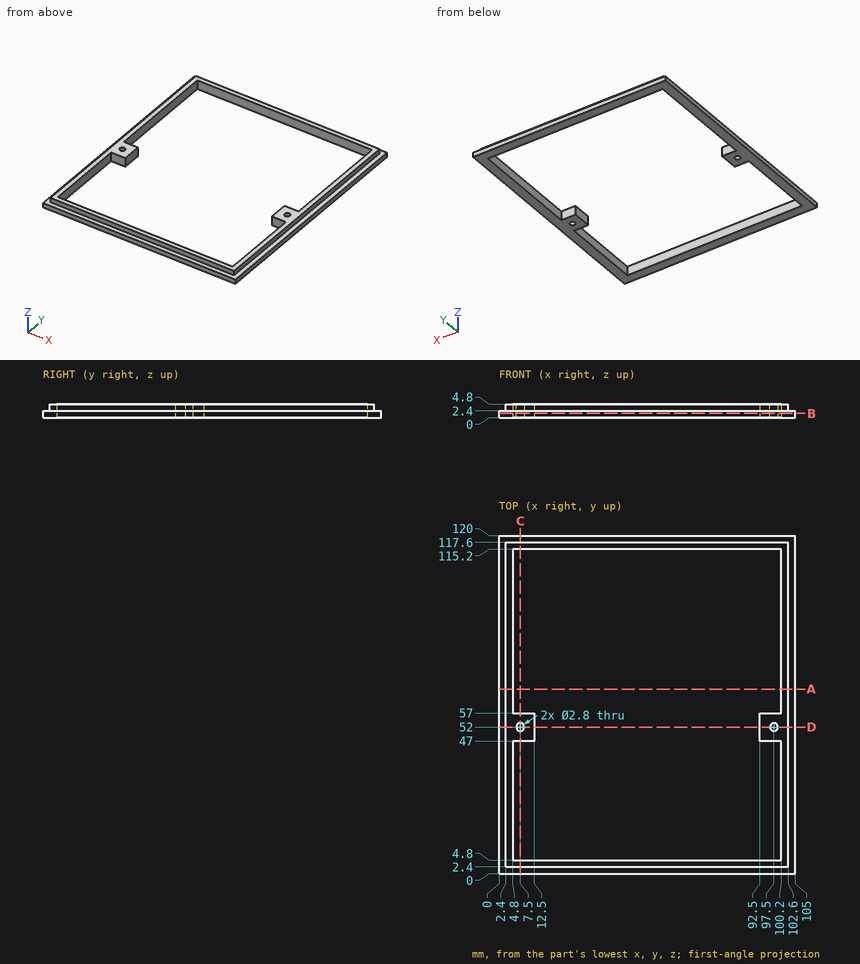
Here's the drawing with two shaded views (mm, measured from the low corner). I have some questions. Coordinates: 2 decimals unless noted, no trailing zeros. Write each loop counter-clockwise with the first axis right and the second up, starting at its lowest first coordinate (ties: lowest second). Pieces come first, ordered by that corner, then holes. Notation, with made-up numbers: M 40,22 L 56,22 A10 ccw 56,26 Z; hole C 18.25,-20.5 d5. An arc over 180 degrees is marked long. Use one line per item in the form item = value.
Q1. If we section it at B-B (z = 1.5): Write out the boundary of the cut face in (x, y), then the cut area to 3 significant figures.
Model answer:
outline = M 0,0 L 105,0 L 105,120 L 0,120 Z; hole M 4.8,4.8 L 100.2,4.8 L 100.2,47 L 92.5,47 L 92.5,57 L 100.2,57 L 100.2,115.2 L 4.8,115.2 L 4.8,57 L 12.5,57 L 12.5,47 L 4.8,47 Z; hole C 7.5,52 d2.8; hole C 97.5,52 d2.8
area = 2,210 mm^2
Q2. If we section it at D-D (y = 52): Write out the boundary of the cut face in (x, z), then the cut area to 3 significant figures.
Model answer:
outline = M 0,0 L 6.1,0 L 6.1,4.8 L 2.4,4.8 L 2.4,2.4 L 0,2.4 Z; M 8.9,0 L 12.5,0 L 12.5,4.8 L 8.9,4.8 Z; M 92.5,0 L 96.1,0 L 96.1,4.8 L 92.5,4.8 Z; M 98.9,0 L 105,0 L 105,2.4 L 102.6,2.4 L 102.6,4.8 L 98.9,4.8 Z
area = 81.6 mm^2
Q3. If we section it at A-A (y = 65.5): Write out the boundary of the cut face in (x, z), then the cut area to 3 significant figures.
Model answer:
outline = M 0,0 L 4.8,0 L 4.8,4.8 L 2.4,4.8 L 2.4,2.4 L 0,2.4 Z; M 100.2,0 L 105,0 L 105,2.4 L 102.6,2.4 L 102.6,4.8 L 100.2,4.8 Z
area = 34.6 mm^2
Q4. If we section it at C-C (x = 7.5): Write out the boundary of the cut face in (y, z).
Model answer:
outline = M 0,0 L 4.8,0 L 4.8,4.8 L 2.4,4.8 L 2.4,2.4 L 0,2.4 Z; M 47,0 L 50.6,0 L 50.6,4.8 L 47,4.8 Z; M 53.4,0 L 57,0 L 57,4.8 L 53.4,4.8 Z; M 115.2,0 L 120,0 L 120,2.4 L 117.6,2.4 L 117.6,4.8 L 115.2,4.8 Z
Q5. For P1, Ø1.4, axis at x = 98, z = 3.5, coming from the -Y side; P2, Ø1.9, axis at y = 38.5, z = 3.5, coming from the -X side; P3, Ø1.9, axis at x = 67, z = 4, coming from the +Y side, each with a flat end and sliding along its axis, tell me the tip position at first contact or that it passes through.
Model answer:
P1 = 2.4
P2 = 2.4
P3 = 117.6
Q6. I need wall thicknesses on line 1 along X through (y, z) = (52, 1.35); line 2 along Y through (x, z) = (7.5, 3.45); line 3 along Y through (x, z) = (97.5, 1.25). Which ranges of each line are inside material? Lowest first, please. Write a range as from..to.
Model answer:
line_1 = 0..6.1, 8.9..12.5, 92.5..96.1, 98.9..105
line_2 = 2.4..4.8, 47..50.6, 53.4..57, 115.2..117.6
line_3 = 0..4.8, 47..50.6, 53.4..57, 115.2..120
